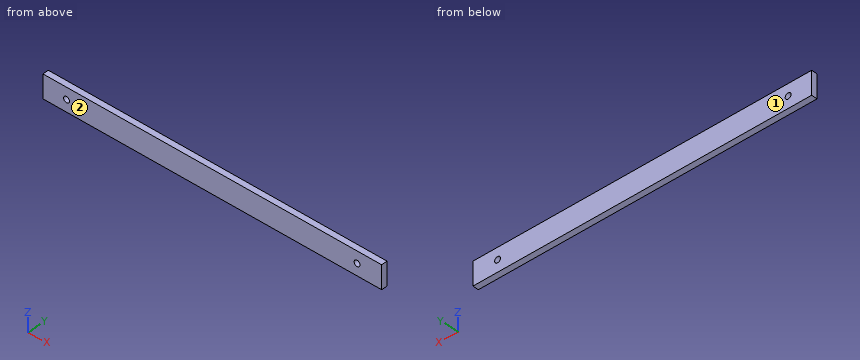
```python
from build123d import *

# Parameters (mm, degrees)
SKETCH1_W           = 365.252
SKETCH1_H           = 25.4
BOSS_EXTRUDE1_DEPTH = 6.35
CUT_EXTRUDE1_REACH  = 368.189
SKETCH2_R           = 3.175


with BuildPart() as part:
    # Sketch1 → Boss-Extrude1 (new body)
    with BuildSketch(Plane(origin=(0, 0, 0), x_dir=(1, 0, 0), z_dir=(0, 1, 0))):
        with Locations((182.626, -12.7)):
            Rectangle(SKETCH1_W, SKETCH1_H)
    extrude(amount=BOSS_EXTRUDE1_DEPTH)

    # Sketch2 → Cut-Extrude1 (cut, up to next)
    with BuildSketch(Plane.XZ, mode=Mode.PRIVATE) as cut_extrude1_sk1:
        with Locations(Location((25.4, 12.7, 0), (0, 0, 270))):
            Circle(SKETCH2_R)
    cut_extrude1_tool1 = extrude(cut_extrude1_sk1.sketch, amount=-CUT_EXTRUDE1_REACH, mode=Mode.PRIVATE) & part.part
    # Sketch2 → Cut-Extrude1 (cut, up to next)
    with BuildSketch(Plane.XZ, mode=Mode.PRIVATE) as cut_extrude1_sk2:
        with Locations(Location((338.738972, 12.7, 0), (0, 0, 270))):
            Circle(SKETCH2_R)
    cut_extrude1_tool2 = extrude(cut_extrude1_sk2.sketch, amount=-CUT_EXTRUDE1_REACH, mode=Mode.PRIVATE) & part.part
    add(cut_extrude1_tool1.solids().sort_by_distance((25.4, 0, 12.7))[0], mode=Mode.SUBTRACT)
    add(cut_extrude1_tool2.solids().sort_by_distance((338.738972, 0, 12.7))[0], mode=Mode.SUBTRACT)


solid = part.part
```
Can you work these out from the model? Positions are in its coordinate system, mm. Face numbers are marked on the shaded views. Round coordinates to 2 decimals unless told otherwise and drop trailing zeros. Order: outer loops, then holes, each group sorted by start corner. A loop starts at its lowest first (then second) coordinate and runs counter-clockwise, first axis right, second up. Notation, with made-up numbers: (68, 45.5) -> (114, 45.5) arc R20 cw to (114, 58.5) -> close; hole circle Ø1 at (-15, -38). An arc over 180 degrees is marked (long way). Return JSON: item names as keys, results as strings. Group by question number.
1. We'd pull the mould along Y, two halves only. Please class the marked faces 1 and 2: released by +Y, released by -Y, zero draft, split by the parting line, or undercut.
2. If we section it at A-A, the plane z = 12.7: Write out the boundary of the cut face in (x, y) (3 decimals), then the cut area to 3 significant figures.
3. If we section it at B-B, the plane x = 25.4: Write out the boundary of the cut face in (y, z) (3 decimals), then the cut area to 3 significant figures.
4. I need wall thicknesses on line 1 (X direction, y = 4.5, z = 12.7) (3 decimals). Which ranges of the line are inside material? Lowest first, please. Write a range as [from, to].
Output values:
{
 "1": {"face 1": "released by +Y", "face 2": "released by -Y"},
 "2": {"outline": "(0, 0) -> (22.225, 0) -> (22.225, 6.35) -> (0, 6.35) -> close; (28.575, 0) -> (335.564, 0) -> (335.564, 6.35) -> (28.575, 6.35) -> close; (341.914, 0) -> (365.252, 0) -> (365.252, 6.35) -> (341.914, 6.35) -> close", "area": "2,240 mm²"},
 "3": {"outline": "(0, 0) -> (6.35, 0) -> (6.35, 9.525) -> (0, 9.525) -> close; (0, 15.875) -> (6.35, 15.875) -> (6.35, 25.4) -> (0, 25.4) -> close", "area": "121 mm²"},
 "4": {"line 1": "[0, 22.225], [28.575, 335.564], [341.914, 365.252]"}
}
